Input: part model. Units: mm. Frame: model coordinates. A direction names the side the tool comes from. Coordinates: 2 decimals unless noted, no trailing zeros. Order: outer loops, then holes, each group sorted by start corner. A loop starts at its lowest first (then second) coordinate and runs counter-clockwise, first axis right, second up. Notation, with made-up numbers: (-0.5, 34) - (56.5, 34) arc R25 cw to (56.5, 46) - close; hole circle Ø2 at (25.25, -4.75). An arc over 180 degrees is marked (long way). One line per question, with ' | ' between items. Start each with the question number.
```python
from build123d import *

# Parameters (mm, degrees)
CROQUIS2_W              = 11.5
CROQUIS2_H              = 37.290106074
SALIENTE_EXTRUIR1_DEPTH = 5
CROQUIS6_W              = 11.5
CROQUIS6_H              = 18.645053037
SALIENTE_EXTRUIR2_DEPTH = 7
CROQUIS4_W              = 1
CROQUIS4_H              = 3
CORTAR_EXTRUIR2_DEPTH   = 6.5
CORTAR_EXTRUIR3_START   = -10.5
CROQUIS5_W              = 2
CROQUIS5_H              = 3
CROQUIS5_W_2            = 3.958309594
CORTAR_EXTRUIR3_DEPTH   = 11.5
CROQUIS7_W              = 8
CROQUIS7_H              = 5
CORTAR_EXTRUIR4_DEPTH   = 15
REDONDEO1_R             = 2


with BuildPart() as part:
    # Croquis2 → Saliente-Extruir1 (new body)
    with BuildSketch(Plane.XY):
        with Locations((-0.75, 0)):
            Rectangle(CROQUIS2_W, CROQUIS2_H)
    extrude(amount=SALIENTE_EXTRUIR1_DEPTH)

    # Croquis2<4> → Cortar-Revolución1 (revolve, cut)
    with BuildSketch(Plane.XY):
        Polygon((-2.5, -18.645053037), (0, -18.645053037), (0, 18.645053037), (-2.5, 18.645053037), (-2.5, 9.645053037), (-3.5, 7), (-3.5, -7), (-2.5, -9.645053037), align=None)
    revolve(axis=Axis((0, 7, 0), (0, 1, 0)), mode=Mode.SUBTRACT)

    # Croquis3 → Cortar-Revolución2 (revolve, cut)
    with BuildSketch(Plane(origin=(0, 0, 0), x_dir=(-1, 0, 0), z_dir=(0, 0, -1))):
        Polygon((0, 0), (0, 3.5), (12, 2.5), (12, 0), align=None)
    revolve(axis=Axis((0, 0, 0), (-1, 0, 0)), mode=Mode.SUBTRACT)

    # Croquis6 → Saliente-Extruir2 (add)
    with BuildSketch(Plane.XY.offset(5)):
        with Locations((-0.75, 9.322526519)):
            Rectangle(CROQUIS6_W, CROQUIS6_H)
    extrude(amount=SALIENTE_EXTRUIR2_DEPTH)

    # Croquis4 → Cortar-Extruir2 (cut)
    with BuildSketch(Plane(origin=(0, 0, 0), x_dir=(-1, 0, 0), z_dir=(0, 0, -1))):
        with Locations((-4.5, 14.145053037)):
            Rectangle(CROQUIS4_W, CROQUIS4_H)
        with Locations((6, 14.145053037)):
            Rectangle(CROQUIS4_W, CROQUIS4_H)
        with Locations((6, -14.145053037)):
            Rectangle(CROQUIS4_W, CROQUIS4_H)
        with Locations((-4.5, -14.145053037)):
            Rectangle(CROQUIS4_W, CROQUIS4_H)
    extrude(amount=-CORTAR_EXTRUIR2_DEPTH, mode=Mode.SUBTRACT)

    # Croquis5 → Cortar-Extruir3 (cut)
    with BuildSketch(Plane(origin=(4, 0, 0), x_dir=(0, 0, -1), z_dir=(1, 0, 0)).offset(CORTAR_EXTRUIR3_START)):
        with Locations((-7.5, 14.145053037)):
            Rectangle(CROQUIS5_W, CROQUIS5_H)
        with Locations((-5.979154797, -14.145053037)):
            Rectangle(CROQUIS5_W_2, CROQUIS5_H)
    extrude(amount=CORTAR_EXTRUIR3_DEPTH, mode=Mode.SUBTRACT)

    # Croquis7 → Cortar-Extruir4 (cut)
    with BuildSketch(Plane(origin=(0, 18.645053037, 0), x_dir=(1, 0, 0), z_dir=(0, 1, 0))):
        with Locations((-0.75, -7.5)):
            Rectangle(CROQUIS7_W, CROQUIS7_H)
    extrude(amount=-CORTAR_EXTRUIR4_DEPTH, mode=Mode.SUBTRACT)

    # Redondeo1
    redondeo1_edges = [part.edges().sort_by_distance(p)[0] for p in [
        (-6.5, -6.322526519, 5),
        (5, -6.322526519, 5),
        (5, 0, 8.5),
        (-6.5, 0, 8.5),
        (5, 9.322526519, 12),
        (-6.5, 9.322526519, 12),
        (-0.75, 0, 12),
        (5, -17.145053037, 5),
        (-6.5, -17.145053037, 5),
    ]]
    fillet(redondeo1_edges, radius=REDONDEO1_R)


solid = part.part
```
(1) Section D-D (x = 0). Output: boundary loops of the cut face in (y, z), then the cut area to 3 significant figures.
(2) Section B-B (z = 9). Output: boundary loops of the cut face in (x, y).
(3) Material intervals for line 1 along Y through (x, z) = (4.5, 3); line 2 along X through (y, z) = (12.5, 9); line 3 along Z through (x, y) = (-4.5, 8), sorted ascending. Write a range as from..to.
(4) Draft query along Y for faces 1 (the face through (-0.7, -12.645, 4.7)), 2 (the face through (-0.8, 18.645, 4.6)), 3 (the face through (-0.1, 14.1, 2.5)), 4 (the face through (-6, 12.645, 5)). Return one class per face: +Y half, -Y half, draft (parallel to the pull), parting line (faces both ways), or undercut.
(5) Pin query (flat end, axial travel): pin 1 (0.8 mm diameter, centred on x = -5, y = 14, fed in from +Z); pin 2 (4 mm diameter, centred on x = -1, z = 8, fed in from -Y); pin 3 (0.9 mm diameter, centred on x = 4.5, y = 13.5, fed in from -Z). Return the tip coordinate at first contact, or that it passes through.
(6) Section A-A (y = 10). Output: boundary loops of the cut face in (x, z), then the cut area to 3 significant figures.
(7) Section C-C (y = 14.5). Output: boundary loops of the cut face in (x, z).
(8) Reachability of faces 5 (the face through (-5.93, -5.22, 4.4)), 6 (the face through (4.3, 12.645, 5.1)), 7 (the face through (4.4, 0.57, 7.33)), 8 (the face through (4, 14, 8.5)) from +Z, -Z, +X, -X, +Y, -Y: full face, straight path, thin tool, end or side. Return the list, or none.
Worked answers:
1) outline: (-18.65, 2.5) - (-9.65, 2.5) - (-7, 3.5) - (7, 3.5) - (9.65, 2.5) - (18.65, 2.5) - (18.65, 5) - (3.65, 5) - (3.65, 10) - (18.65, 10) - (18.65, 12) - (2, 12) arc R2 ccw to (0, 10) - (0, 5) - (-12.65, 5) - (-12.65, 4) - (-15.65, 4) - (-15.65, 5) - (-18.65, 5) - close | area: 128 mm²
2) outline: (-6.5, 2) arc R2 ccw to (-4.5, 0) - (3, 0) arc R2 ccw to (5, 2) - (5, 18.65) - (3.25, 18.65) - (3.25, 3.65) - (-4.75, 3.65) - (-4.75, 18.65) - (-6.5, 18.65) - close
3) line 1: y = -18.65..-15.65, -12.65..12.65, 15.65..18.65 | line 2: x = -6.5..-4.75, 3.25..5 | line 3: z = 0..5, 10..12
4) face 1: undercut | face 2: +Y half | face 3: draft | face 4: undercut
5) pin 1: stops at z = 12 | pin 2: stops at y = 0 | pin 3: stops at z = 8.5
6) outline: (-6.5, 0) - (-2.5, 0) arc R2.5 cw to (2.5, 0) - (5, 0) - (5, 10) arc R2 ccw to (3, 12) - (-4.5, 12) arc R2 ccw to (-6.5, 10) - close; hole (-4.75, 5) - (3.25, 5) - (3.25, 10) - (-4.75, 10) - close | area: 86.5 mm²
7) outline: (-6.5, 8.5) - (-4.75, 8.5) - (-4.75, 10) - (3.25, 10) - (3.25, 8.5) - (5, 8.5) - (5, 10) arc R2 ccw to (3, 12) - (-4.5, 12) arc R2 ccw to (-6.5, 10) - close; (-5.5, 0) - (-2.5, 0) arc R2.5 cw to (2.5, 0) - (4, 0) - (4, 6.5) - (3.25, 6.5) - (3.25, 5) - (-4.75, 5) - (-4.75, 6.5) - (-5.5, 6.5) - close
8) face 5: +Z, -X, -Y | face 6: +X | face 7: +Z, +X, -Y | face 8: +X, -X
